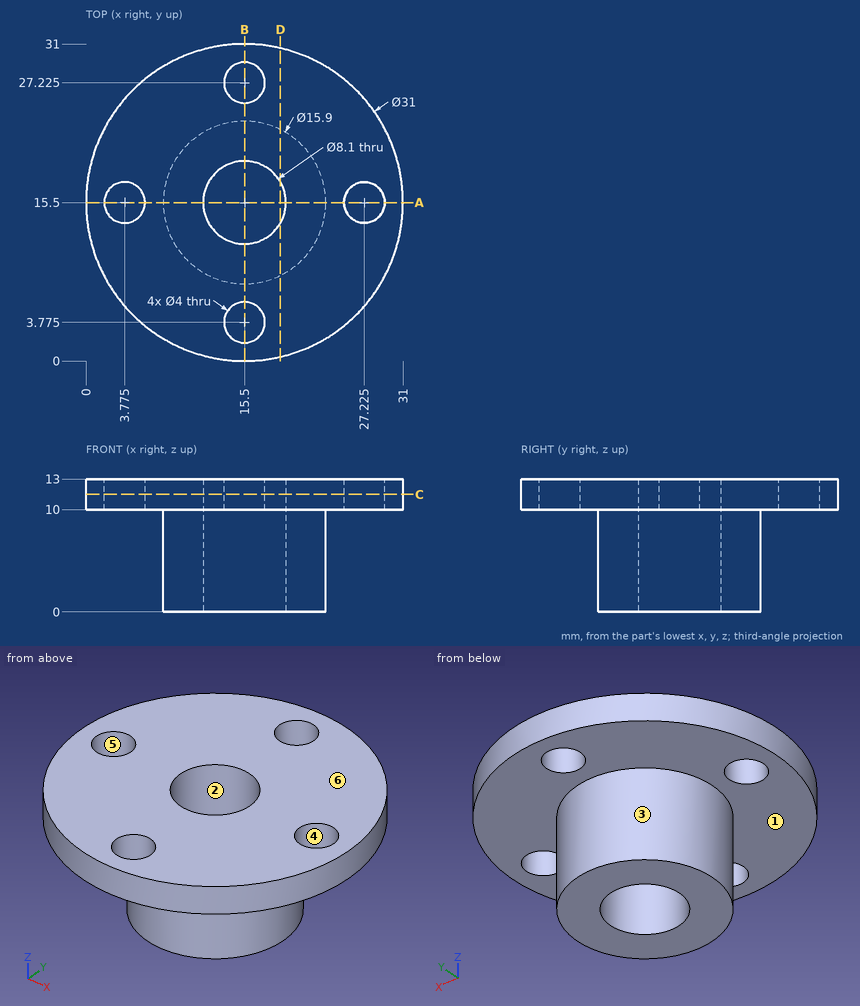
Here's the drawing with two shaded views (mm, measured from the low corner). I have some questions. A direction names the side the tool comes from. Coordinates: 2 decimals unless noted, no trailing zeros. Loops run counter-clockwise (first coordinate to the right, second up) from the corner with the lowest first, then second, coordinate; pieces in that order, holes last.
Item 1: Suppose I cut it at D-D (x = 19). Please give me the cut outline in (y, z), then the cut area to 3 significant figures.
Answers below:
outline: (0.4, 10) - (8.36, 10) - (8.36, 0) - (13.46, 0) - (13.46, 13) - (0.4, 13) - close; (17.54, 0) - (22.64, 0) - (22.64, 10) - (30.6, 10) - (30.6, 13) - (17.54, 13) - close
area: 180 mm2
Item 2: Suppose I cut it at C-C (z = 11.5). Please give me the cut outline in (x, y) (3 decimals), then the cut area to 3 significant figures.
Answers below:
outline: circle Ø31 at (15.5, 15.5); hole circle Ø4 at (3.775, 15.5); hole circle Ø8.1 at (15.5, 15.5); hole circle Ø4 at (15.5, 3.775); hole circle Ø4 at (15.5, 27.225); hole circle Ø4 at (27.225, 15.5)
area: 653 mm2
Item 3: Which directions (+Z, -Z, +X, -X, +Y, -Y) give clear straight access to the entire face, cutting with the end or side of a thin tool? Please do the marked faces 1 and 2.
Answers below:
face 1: -Z
face 2: +Z, -Z
Item 4: Suppose I cut it at A-A (y = 15.5). Please give me the cut outline in (x, z) (3 decimals).
Answers below:
outline: (0, 10) - (1.775, 10) - (1.775, 13) - (0, 13) - close; (5.775, 10) - (7.55, 10) - (7.55, 0) - (11.45, 0) - (11.45, 13) - (5.775, 13) - close; (19.55, 0) - (23.45, 0) - (23.45, 10) - (25.225, 10) - (25.225, 13) - (19.55, 13) - close; (29.225, 10) - (31, 10) - (31, 13) - (29.225, 13) - close
Item 5: If we mould it in two halves opening along X, with no side actions, what happens to the marked faces 3, 4, 5 and 6? For each: released by +X, released by -X, zero draft, split by the parting line, or undercut.
Answers below:
face 3: split by the parting line
face 4: undercut
face 5: undercut
face 6: zero draft
Item 6: Please list where these lines run through material, in increasing order: L1, parallel to Z at x = 5.5, y = 5.5; L2, parallel to X at y = 17, z = 8.25; L3, parallel to X at y = 13, z = 6.5.
Answers below:
L1: z = 10 to 13
L2: x = 7.69 to 11.74, 19.26 to 23.31
L3: x = 7.95 to 12.31, 18.69 to 23.05
Item 7: I'm going to push flat-ended pins straight in: pin 1 (5 mm diameter, centred on x = 22.5, y = 25.5, fed in from -Z); pin 2 (4 mm diameter, centred on x = 17.5, z = 4.5, fed in from -Y); pin 3 (2 mm diameter, centred on y = 13.5, z = 10.5, fed in from -X). Where does each tip first touch, or does it pass through?
Answers below:
pin 1: stops at z = 10
pin 2: stops at y = 7.55
pin 3: stops at x = 0.03
